Verification items for the finished model (mm, model axes). Face numbers are marked on the shaded views. A direction names the side the tool comes from. Coordinates: 2 decimals unless noted, no trailing zeros. Order: outer loops, then holes, each group sorted by start corner. A loop starts at its lowest first (then second) coordinate and runs counter-clockwise, first axis right, second up. Notation, with made-up numbers: (18, -23.75) -> (71, -23.75) arc R34 ccw to (71, 10.25) -> close; hole circle Ø3 at (-5.75, 22.25). An arc over 180 degrees is marked (long way). Write item = value, one per line. Start each with the question number.
1. Cross-section at B-B on y = -33. Record the cut outline in (x, z) (3 decimals).
2. Thickness scan on line 1 along Y through (x, z) = (-10.5, 5.5); line 2 along Y through (x, z) = (8.5, 0); line 3 along Y through (x, z) = (30.5, -32). Record the ranges inside material, lowest first. Write a range as from..to.
3. Cross-section at A-A on x = -32. Record the cut outline in (y, z) (3 decimals), plus the area to 3 significant figures.
4. Set-up check for the marked faces 1, 2 and 3: record each of +Z, -Z, +X, -X, +Y, -Y from which the full face is reachable in a straight line by a thin tool's end or side.
5. Go/stop test with flat-tipped pins: P1, Ø1.3, axis at y = -33, z = 8, coming from the -X side; P2, Ø10, axis at y = -6.5, z = 1.5, coming from the +X side; P3, Ø6, axis at x = -22.5, y = -20.5, coming from the +Z side. Record where each tip stops, or that it passes through.
6. Release check for a two-part mould opening along Y. For the marked faces 4, 5, 6 and 7 record: +Y half, -Y half, draft (parallel to the pull), parting line (faces both ways), or undercut.
7. Cross-section at C-C on z = -4. Give the number of separate pieces and of enclosed holes in the cut face, plus the area to 3 significant figures.
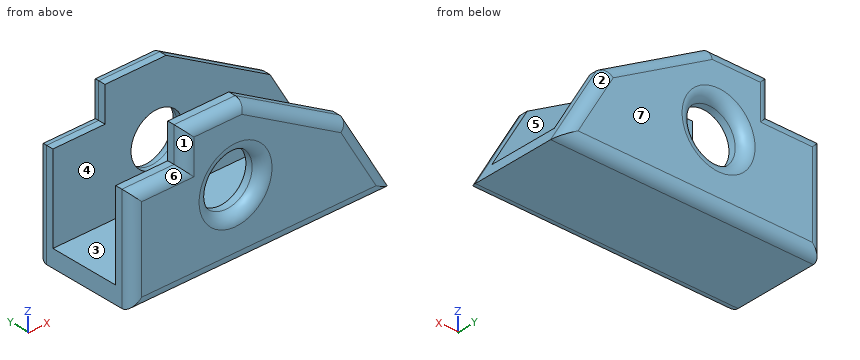
from build123d import *

# Parameters (mm, degrees)
F1_DEPTH = 38.1
F3_D     = 19.05
F4_W     = 19.05
F4_H     = 12.7
F5_DEPTH = 38.101
F6_W     = 25.4
F6_H     = 50.8172035844
F7_DEPTH = 52.1778825103
F8_DEPTH = 43.9057145722
F9_R     = 3.81
F10_R    = 3.81


with BuildPart() as f1:
    # F0 (on Front) → F1 (new body)
    with BuildSketch(Plane.XZ):
        Polygon((-10.7748825103, 15.1617240763), (-52.1768825103, 15.1617240763), (-52.1768825103, -35.6382759237), (43.9047145722, -35.6382759237), (27.2504226012, -6.7921960659), align=None)
    extrude(amount=F1_DEPTH)

    # F3 (through all)
    with Locations(Plane(origin=(0, 0, 0), x_dir=(1, 0, 0), z_dir=(0, 1, 0))):
        with Locations((-14.0768825103, 10.2382759237)):
            Hole(F3_D / 2)

    # F4 (on face) → F5 (cut, through all)
    with BuildSketch(Plane.XZ.offset(38.1)):
        with Locations((-42.6518825103, 8.8117240763)):
            Rectangle(F4_W, F4_H)
    extrude(amount=-F5_DEPTH, mode=Mode.SUBTRACT)

    # F6 (on Right) → F7 (cut, through all)
    with BuildSketch(Plane.YZ):
        with Locations((-19.05, -3.8796741316)):
            Rectangle(F6_W, F6_H)
    extrude(amount=-F7_DEPTH, mode=Mode.SUBTRACT)

    # F8 (cut, through all): a face of the model
    f8_faces = [f1.faces().sort_by_distance(p)[0] for p in [
        (0, -19.05, -10.1737165826),
    ]]
    extrude(f8_faces, amount=-F8_DEPTH, mode=Mode.SUBTRACT)

    # F9
    f9_edges = [f1.edges().sort_by_distance(p)[0] for p in [
        (8.23777, -38.1, 4.184764),
        (35.577569, -38.1, -21.215236),
        (-4.136084, -38.1, -35.638276),
        (-52.176883, -38.1, -16.588276),
        (-42.651883, -38.1, 2.461724),
        (-33.126883, -38.1, 8.811724),
        (-21.950883, -38.1, 15.161724),
        (-23.601883, -38.1, -10.238276),
    ]]
    fillet(f9_edges, radius=F9_R)

    # F10
    f10_edges = [f1.edges().sort_by_distance(p)[0] for p in [
        (8.23777, 0, 4.184764),
        (35.577569, 0, -21.215236),
        (-4.136084, 0, -35.638276),
        (-52.176883, 0, -16.588276),
        (-42.651883, 0, 2.461724),
        (-33.126883, 0, 8.811724),
        (-21.950883, 0, 15.161724),
        (-23.601883, 0, -10.238276),
    ]]
    fillet(f10_edges, radius=F10_R)


solid = f1.part
Worked out:
q1.outline = (-52.177, -35.638) -> (43.905, -35.638) -> (27.25, -6.792) -> (-10.775, 15.162) -> (-33.127, 15.162) -> (-33.127, 2.462) -> (-52.177, 2.462) -> close; hole circle Ø19.05 at (-14.077, -10.238)
q2.line_1 = -38.1..-31.75, -6.35..0
q2.line_2 = -38.09..-31.75, -6.35..-0.01
q2.line_3 = -38.1..0
q3.outline = (-38.1, -31.828) arc R3.81 ccw to (-34.29, -35.638) -> (-3.81, -35.638) arc R3.81 ccw to (0, -31.828) -> (0, -1.348) arc R3.81 ccw to (-1.105, 1.335) -> (-1.105, 14.035) arc R3.81 ccw to (-3.81, 15.162) -> (-6.35, 15.162) -> (-6.35, -29.288) -> (-31.75, -29.288) -> (-31.75, 15.162) -> (-34.29, 15.162) arc R3.81 ccw to (-36.995, 14.035) -> (-36.995, 1.335) arc R3.81 ccw to (-38.1, -1.348) -> close
q3.area = 766 mm²
q4.face_1 = +Z, -X, -Y
q4.face_2 = +Z, +X, +Y
q4.face_3 = +Z, +X, -X
q5.P1 = -33.13
q5.P2 = 21.54
q5.P3 = -29.29
q6.face_4 = undercut
q6.face_5 = undercut
q6.face_6 = -Y half
q6.face_7 = +Y half
q7.separate_pieces = 4
q7.enclosed_holes = 0
q7.area = 730 mm²
